Model file for the job. Use its own axes, mm. A direction names the side the tool comes from. Give positions to 0.01 mm unless a question says otherwise; leave off trailing zeros. Write each loop counter-clockwise with the first axis right and the second up, starting at its lowest first coordinate (ties: lowest second). Pieces come first, ordered by that corner, then holes.
```python
from build123d import *

# Parameters (mm, degrees)
SKETCH1_R           = 250
BOSS_EXTRUDE1_DEPTH = 80
SHELL1_T            = -1.2
SKETCH2_R           = 7.5
CUT_EXTRUDE1_DEPTH  = 10


with BuildPart() as part:
    # Sketch1 → Boss-Extrude1 (new body)
    with BuildSketch(Plane.XY):
        Circle(SKETCH1_R)
    extrude(amount=BOSS_EXTRUDE1_DEPTH)

    # Shell1
    shell1_openings = [part.faces().sort_by_distance(p)[0] for p in [
        (0, 0, 0),
    ]]
    offset(amount=SHELL1_T, openings=shell1_openings, kind=Kind.INTERSECTION)

    # Sketch2 → Cut-Extrude1 (cut)
    with BuildSketch(Plane(origin=(0, 0, 78.8), x_dir=(-1, 0, 0), z_dir=(0, 0, -1))):
        Circle(SKETCH2_R)
    extrude(amount=-CUT_EXTRUDE1_DEPTH, mode=Mode.SUBTRACT)


solid = part.part
```
1. Slice it at D-D, the plane y = 83. Write the cut outline in (x, z).
Calculated:
outline: (-235.82, 0) - (-234.55, 0) - (-234.55, 78.8) - (234.55, 78.8) - (234.55, 0) - (235.82, 0) - (235.82, 80) - (-235.82, 80) - close
2. Which spindle directions (+Z, -Z, +X, -X, +Y, -Y) get a long thin tool onto all of the face, cutting with end or side? Do faces 1 (the flat face through (-3, -52, 78.8)), 2 (the cylindrical face through (7.493, 0.33, 79.392)). Say none if no direction does.
Calculated:
face 1: -Z
face 2: +Z, -Z
3. Pull direction X, two halves, no side cores. Call faces 3 (the cylindrical face through (-53.935, -242.884, 38.848)), 4 (the flat face through (-3, -52, 80)), 5 (the cylindrical face through (-249.76, 10.99, 39.44)): +X half, -X half, draft (parallel to the pull), parting line (faces both ways), or undercut.
Calculated:
face 3: undercut
face 4: draft
face 5: parting line
4. Probe probe 1 along Y at (x, z) = (0, 79.3); probe 2 along Y at (x, z) = (0, 61); probe 3 along X at (y, z) = (114, 59). List the from-to ranges inside material, lowest first.
Calculated:
probe 1: y = -250 to -7.5, 7.5 to 250
probe 2: y = -250 to -248.8, 248.8 to 250
probe 3: x = -222.49 to -221.15, 221.15 to 222.49
5. Pin check, flat tips, straight feed: P1, Ø6, axis at x = -111, y = -107, coming from the -Z side; P2, Ø3, axis at x = -101.5, z = 35.5, coming from the +Y side; P3, Ø8, axis at y = -67.5, z = 64, coming from the -X side; P4, Ø13.5, axis at x = 0, y = 0, coming from the +Z side. Stop position of each tip, or through.
Calculated:
P1: stops at z = 78.8
P2: stops at y = 229.13
P3: stops at x = -241.8
P4: passes through
6. Slice it at C-C, the plane z = 64. Write the cut outline in (x, y).
Calculated:
outline: circle Ø500 at (0, 0); hole circle Ø497.6 at (0, 0)
7. Slice it at A-A, the plane x = 0. Write the cut outline in (y, z), and give its area (3 significant figures).
Calculated:
outline: (-250, 0) - (-248.8, 0) - (-248.8, 78.8) - (-7.5, 78.8) - (-7.5, 80) - (-250, 80) - close; (7.5, 78.8) - (248.8, 78.8) - (248.8, 0) - (250, 0) - (250, 80) - (7.5, 80) - close
area: 771 mm2
